```python
from build123d import *

# Parameters (mm, degrees)
F0_W     = 2
F0_H     = 2
F1_DEPTH = 96
F2_R     = 0.5
F3_DEPTH = 48
F4_START = 92
F4_DEPTH = 6
F5_START = 94
F0_H_2   = 44
F5_DEPTH = 2
F6_R     = 0.25
F7_DEPTH = 0.5
F8_R     = 0.25
F9_DEPTH = 0.5


with BuildPart() as f1:
    # F0 (on Top) → F1 (new body)
    with BuildSketch(Plane.XY):
        with Locations((-44.9200854897, -5.6579317451)):
            Rectangle(F0_W, F0_H)
    extrude(amount=F1_DEPTH)



with BuildPart() as f1b:
    # F0 (on Top) → F1, piece 2 (new body)
    with BuildSketch(Plane.XY):
        with Locations((1.0799145103, -5.6579317451)):
            Rectangle(F0_W, F0_H)
    extrude(amount=F1_DEPTH)


with BuildPart() as f1_1:
    add(f1.part)

    add(f1b.part)  # F3 merges F1b
    # F2 (on face) → F3 (join)
    with BuildSketch(Plane(origin=(-45.9200854897, 0, 0), x_dir=(0, -1, 0), z_dir=(-1, 0, 0))):
        with Locations((5.6579317451, 95)):
            Circle(F2_R)
    extrude(amount=-F3_DEPTH)



with BuildPart() as f4:
    # F0 (on Top) → F4 (new body)
    with BuildSketch(Plane.XY.offset(F4_START)):
        Polygon((-1.9200854897, 41.3420682549), (0.0799145103, 41.3420682549), (2.0799145103, 41.3420682549), (4.0799145103, 41.3420682549), (4.0799145103, 41.5920682549), (-1.9200854897, 41.5920682549), align=None)
    extrude(amount=F4_DEPTH)


with BuildPart() as f4b:
    # F0 (on Top) → F4, piece 2 (new body)
    with BuildSketch(Plane.XY.offset(F4_START)):
        Polygon((-47.9200854897, 41.3420682549), (-45.9200854897, 41.3420682549), (-43.9200854897, 41.3420682549), (-41.9200854897, 41.3420682549), (-41.9200854897, 41.5920682549), (-47.9200854897, 41.5920682549), align=None)
    extrude(amount=F4_DEPTH)


with BuildPart() as f1_2:
    add(f1_1.part)

    add(f4.part)  # F5 merges F4

    add(f4b.part)  # F5 merges F4b
    # F0 (on Top) → F5 (join)
    with BuildSketch(Plane.XY.offset(F5_START)):
        with Locations((-44.9200854897, -3.6579317451)):
            Rectangle(F0_W, F0_H)
        with Locations((1.0799145103, -3.6579317451)):
            Rectangle(F0_W, F0_H)
        with Locations((-44.9200854897, 19.3420682549)):
            Rectangle(F0_W, F0_H_2)
        with Locations((1.0799145103, 19.3420682549)):
            Rectangle(F0_W, F0_H_2)
    extrude(amount=F5_DEPTH)

    # F6 (on face) → F7 (cut)
    with BuildSketch(Plane(origin=(0, 41.5920682549, 0), x_dir=(-1, 0, 0), z_dir=(0, 1, 0))):
        with Locations((46.9200854897, 97)):
            Circle(F6_R)
        with Locations((42.9200854897, 97)):
            Circle(F6_R)
        with Locations((42.9200854897, 93)):
            Circle(F6_R)
        with Locations((46.9200854897, 93)):
            Circle(F6_R)
    extrude(amount=-F7_DEPTH, mode=Mode.SUBTRACT)

    # F8 (on face) → F9 (cut)
    with BuildSketch(Plane(origin=(0, 41.5920682549, 0), x_dir=(-1, 0, 0), z_dir=(0, 1, 0))):
        with Locations((-3.0799145103, 97)):
            Circle(F8_R)
        with Locations((0.9200854897, 97)):
            Circle(F8_R)
        with Locations((0.9200854897, 93)):
            Circle(F8_R)
        with Locations((-3.0799145103, 93)):
            Circle(F8_R)
    extrude(amount=-F9_DEPTH, mode=Mode.SUBTRACT)


solid = f1_2.part
```
The model under review builds one solid part; all positions refer to its coordinate system, in mm. A direction names the side the tool comes from. Give positions to 0.01 mm unless a question says otherwise; leave off trailing zeros. Write each loop counter-clockwise with the first axis right and the second up, starting at its lowest first coordinate (ties: lowest second). Pieces come first, ordered by that corner, then holes. Notation, with made-up numbers: M 41.25,-19 L 70.25,-19 A18 cw 70.25,-14 Z; hole C 7,39 d8. An arc over 180 degrees is marked long. Write each question's results on one line, items separated by ' | '. Start each with the question number.
1. Mouldability with a two-part tool opening along Y and no side actions: class faces 5 (the flat face through (1, 19, 94)), 6 (the flat face through (-45, -6.658, 47)), 7 (the flat face through (-45.92, -6, 48)), 8 (the flat face through (1, 41.592, 95)) as released by +Y, released by -Y, zero draft, split by the parting line, or undercut.
2. We need section B-B (y = 16). Write out the cut boundary in (x, z), and give its area (3 significant figures).
3. For probe 1 along X at (y, z) = (41.4, 93); probe 2 along Y at (x, z) = (1.5, 49), list the stretches that pass through material, from the lowest coordinate up. Write a range as [from, to].
4. Insertion check: pin 1 Ø1 at (x, z) = (1, 65) entering from +Y; pin 2 Ø1 at (x, y) = (-41.5, 33.5) entering from +Z; pin 3 Ø2 at (x, y) = (-45, 29.5) entering from -Z; pin 4 Ø1 at (x, y) = (-45.5, 22.5) entering from +Z. Each pin has a flat end and moves straight along its axis. Give the tip position at first contact, or say it passes through.
5. We need section A-A (z = 72). Write out the cut boundary in (x, y).
6. We need section C-C (x = -19.5). Write out the cut boundary in (y, z), and give its area (3 significant figures).
7. For faces 1 (the flat face through (-45, 41.342, 93.6)), 2 (the flat face through (-45, -6, 0)), 3 (the flat face through (1, 18, 96)), 4 (the flat face through (-45, 19, 94)), list the 3-axis set-ups (+Z, -Z, +X, -X, +Y, -Y) from which the entire face can be reached by the end or side of a thin tool; tool diameter is ignored.
Results found:
1) face 5: undercut | face 6: released by -Y | face 7: zero draft | face 8: released by +Y
2) outline: M -45.92,94 L -43.92,94 L -43.92,96 L -45.92,96 Z; M 0.08,94 L 2.08,94 L 2.08,96 L 0.08,96 Z | area: 8.00 mm^2
3) probe 1: x = [-47.92, -47.17], [-46.67, -43.17], [-42.67, -41.92], [-1.92, -1.17], [-0.67, 2.83], [3.33, 4.08] | probe 2: y = [-6.66, -4.66]
4) pin 1: stops at y = -4.66 | pin 2: passes through | pin 3: stops at z = 94 | pin 4: stops at z = 96
5) outline: M -45.92,-6.66 L -43.92,-6.66 L -43.92,-4.66 L -45.92,-4.66 Z; M 0.08,-6.66 L 2.08,-6.66 L 2.08,-4.66 L 0.08,-4.66 Z
6) outline: C -5.66,95 d1 | area: 0.785 mm^2
7) face 1: none | face 2: -Z, +X, -X, +Y, -Y | face 3: +Z, +X, -X, -Y | face 4: -Z, +X, -X
